from build123d import *

# Parameters (mm, degrees)
EXTRUDE_1_DEPTH = 50


with BuildPart() as part:
    # 草图1 → 凸台-拉伸1 (new body)
    with BuildSketch(Plane(origin=(0, 0, 0), x_dir=(0, 0, -1), z_dir=(1, 0, 0))):
        with BuildLine():
            Line((-5.14957074, -13.70467014), (-4.14957074, -13.70467014))
            Line((-4.14957074, -13.70467014), (-4.14957074, -12.70467014))
            Line((-4.14957074, -12.70467014), (-8.29957074, -12.70467014))
            Line((-8.29957074, -12.70467014), (-8.29957074, -9.3688837))
            Line((-8.29957074, -9.3688837), (-4.43535718, -5.50467014))
            Line((-4.43535718, -5.50467014), (4.3362157, -5.50467014))
            Line((4.3362157, -5.50467014), (8.20042926, -9.3688837))
            Line((8.20042926, -9.3688837), (8.20042926, -12.70467014))
            Line((8.20042926, -12.70467014), (4.05042926, -12.70467014))
            Line((4.05042926, -12.70467014), (4.05042926, -13.70467014))
            Line((4.05042926, -13.70467014), (5.05042926, -13.70467014))
            Line((5.05042926, -13.70467014), (5.05042926, -14.70467014))
            Line((5.05042926, -14.70467014), (12.45042926, -14.70467014))
            ThreePointArc((12.45042926, -14.70467014), (14.218196213, -13.972437093), (14.95042926, -12.20467014))
            Line((14.95042926, -12.20467014), (14.95042926, -4.80467014))
            Line((14.95042926, -4.80467014), (13.95042926, -4.80467014))
            Line((13.95042926, -4.80467014), (13.95042926, -3.80467014))
            Line((13.95042926, -3.80467014), (12.95042926, -3.80467014))
            Line((12.95042926, -3.80467014), (12.95042926, -7.95467014))
            Line((12.95042926, -7.95467014), (9.61464282, -7.95467014))
            Line((9.61464282, -7.95467014), (5.75042926, -4.09045658))
            Line((5.75042926, -4.09045658), (5.75042926, 4.6811163))
            Line((5.75042926, 4.6811163), (9.61464282, 8.54532986))
            Line((9.61464282, 8.54532986), (12.95042926, 8.54532986))
            Line((12.95042926, 8.54532986), (12.95042926, 4.39532986))
            Line((12.95042926, 4.39532986), (13.95042926, 4.39532986))
            Line((13.95042926, 4.39532986), (13.95042926, 5.39532986))
            Line((13.95042926, 5.39532986), (14.95042926, 5.39532986))
            Line((14.95042926, 5.39532986), (14.95042926, 12.79532986))
            ThreePointArc((14.95042926, 12.79532986), (14.218196213, 14.563096813), (12.45042926, 15.29532986))
            Line((12.45042926, 15.29532986), (5.05042926, 15.29532986))
            Line((5.05042926, 15.29532986), (5.05042926, 14.29532986))
            Line((5.05042926, 14.29532986), (4.05042926, 14.29532986))
            Line((4.05042926, 14.29532986), (4.05042926, 13.29532986))
            Line((4.05042926, 13.29532986), (8.20042926, 13.29532986))
            Line((8.20042926, 13.29532986), (8.20042926, 9.95954342))
            Line((8.20042926, 9.95954342), (4.3362157, 6.09532986))
            Line((4.3362157, 6.09532986), (-4.43535718, 6.09532986))
            Line((-4.43535718, 6.09532986), (-8.29957074, 9.95954342))
            Line((-8.29957074, 9.95954342), (-8.29957074, 13.29532986))
            Line((-8.29957074, 13.29532986), (-4.14957074, 13.29532986))
            Line((-4.14957074, 13.29532986), (-4.14957074, 14.29532986))
            Line((-4.14957074, 14.29532986), (-5.14957074, 14.29532986))
            Line((-5.14957074, 14.29532986), (-5.14957074, 15.29532986))
            Line((-5.14957074, 15.29532986), (-12.54957074, 15.29532986))
            ThreePointArc((-12.54957074, 15.29532986), (-14.317337693, 14.563096813), (-15.04957074, 12.79532986))
            Line((-15.04957074, 12.79532986), (-15.04957074, 5.39532986))
            Line((-15.04957074, 5.39532986), (-14.04957074, 5.39532986))
            Line((-14.04957074, 5.39532986), (-14.04957074, 4.39532986))
            Line((-14.04957074, 4.39532986), (-13.04957074, 4.39532986))
            Line((-13.04957074, 4.39532986), (-13.04957074, 8.54532986))
            Line((-13.04957074, 8.54532986), (-9.7137843, 8.54532986))
            Line((-9.7137843, 8.54532986), (-5.84957074, 4.6811163))
            Line((-5.84957074, 4.6811163), (-5.84957074, -4.09045658))
            Line((-5.84957074, -4.09045658), (-9.7137843, -7.95467014))
            Line((-9.7137843, -7.95467014), (-13.04957074, -7.95467014))
            Line((-13.04957074, -7.95467014), (-13.04957074, -3.80467014))
            Line((-13.04957074, -3.80467014), (-14.04957074, -3.80467014))
            Line((-14.04957074, -3.80467014), (-14.04957074, -4.80467014))
            Line((-14.04957074, -4.80467014), (-15.04957074, -4.80467014))
            Line((-15.04957074, -4.80467014), (-15.04957074, -12.20467014))
            ThreePointArc((-15.04957074, -12.20467014), (-14.317337693, -13.972437093), (-12.54957074, -14.70467014))
            Line((-12.54957074, -14.70467014), (-5.14957074, -14.70467014))
            Line((-5.14957074, -14.70467014), (-5.14957074, -13.70467014))
        make_face()
        with BuildLine():
            Line((-10.04957074, 9.79532986), (-13.04957074, 9.79532986))
            ThreePointArc((-13.04957074, 9.79532986), (-13.403124131, 9.941776469), (-13.54957074, 10.29532986))
            Line((-13.54957074, 10.29532986), (-13.54957074, 13.29532986))
            ThreePointArc((-13.54957074, 13.29532986), (-13.403124131, 13.648883251), (-13.04957074, 13.79532986))
            Line((-13.04957074, 13.79532986), (-10.04957074, 13.79532986))
            ThreePointArc((-10.04957074, 13.79532986), (-9.696017349, 13.648883251), (-9.54957074, 13.29532986))
            Line((-9.54957074, 13.29532986), (-9.54957074, 10.29532986))
            ThreePointArc((-9.54957074, 10.29532986), (-9.696017349, 9.941776469), (-10.04957074, 9.79532986))
        make_face(mode=Mode.SUBTRACT)
        with BuildLine():
            Line((-10.04957074, -13.20467014), (-13.04957074, -13.20467014))
            ThreePointArc((-13.04957074, -13.20467014), (-13.403124131, -13.058223531), (-13.54957074, -12.70467014))
            Line((-13.54957074, -12.70467014), (-13.54957074, -9.70467014))
            ThreePointArc((-13.54957074, -9.70467014), (-13.403124131, -9.351116749), (-13.04957074, -9.20467014))
            Line((-13.04957074, -9.20467014), (-10.04957074, -9.20467014))
            ThreePointArc((-10.04957074, -9.20467014), (-9.696017349, -9.351116749), (-9.54957074, -9.70467014))
            Line((-9.54957074, -9.70467014), (-9.54957074, -12.70467014))
            ThreePointArc((-9.54957074, -12.70467014), (-9.696017349, -13.058223531), (-10.04957074, -13.20467014))
        make_face(mode=Mode.SUBTRACT)
        with BuildLine():
            Line((12.95042926, 9.79532986), (9.95042926, 9.79532986))
            ThreePointArc((9.95042926, 9.79532986), (9.596875869, 9.941776469), (9.45042926, 10.29532986))
            Line((9.45042926, 10.29532986), (9.45042926, 13.29532986))
            ThreePointArc((9.45042926, 13.29532986), (9.596875869, 13.648883251), (9.95042926, 13.79532986))
            Line((9.95042926, 13.79532986), (12.95042926, 13.79532986))
            ThreePointArc((12.95042926, 13.79532986), (13.303982651, 13.648883251), (13.45042926, 13.29532986))
            Line((13.45042926, 13.29532986), (13.45042926, 10.29532986))
            ThreePointArc((13.45042926, 10.29532986), (13.303982651, 9.941776469), (12.95042926, 9.79532986))
        make_face(mode=Mode.SUBTRACT)
        with BuildLine():
            Line((13.45042926, -9.70467014), (13.45042926, -12.70467014))
            ThreePointArc((13.45042926, -12.70467014), (13.303982651, -13.058223531), (12.95042926, -13.20467014))
            Line((12.95042926, -13.20467014), (9.95042926, -13.20467014))
            ThreePointArc((9.95042926, -13.20467014), (9.596875869, -13.058223531), (9.45042926, -12.70467014))
            Line((9.45042926, -12.70467014), (9.45042926, -9.70467014))
            ThreePointArc((9.45042926, -9.70467014), (9.596875869, -9.351116749), (9.95042926, -9.20467014))
            Line((9.95042926, -9.20467014), (12.95042926, -9.20467014))
            ThreePointArc((12.95042926, -9.20467014), (13.303982651, -9.351116749), (13.45042926, -9.70467014))
        make_face(mode=Mode.SUBTRACT)
        with BuildLine():
            Line((-4.07998961, 3.61864195), (-3.37288283, 4.32574873))
            Line((-3.37288283, 4.32574873), (-2.07404174, 3.02690764))
            ThreePointArc((-2.07404174, 3.02690764), (-0.04957074, 3.69532986), (1.97490026, 3.02690764))
            Line((1.97490026, 3.02690764), (3.27374135, 4.32574873))
            Line((3.27374135, 4.32574873), (3.98084813, 3.61864195))
            Line((3.98084813, 3.61864195), (2.68200704, 2.31980086))
            ThreePointArc((2.68200704, 2.31980086), (3.35042926, 0.29532986), (2.68200704, -1.72914114))
            Line((2.68200704, -1.72914114), (3.98084813, -3.02798223))
            Line((3.98084813, -3.02798223), (3.27374135, -3.73508901))
            Line((3.27374135, -3.73508901), (1.97490026, -2.43624792))
            ThreePointArc((1.97490026, -2.43624792), (-0.04957074, -3.10467014), (-2.07404174, -2.43624792))
            Line((-2.07404174, -2.43624792), (-3.37288283, -3.73508901))
            Line((-3.37288283, -3.73508901), (-4.07998961, -3.02798223))
            Line((-4.07998961, -3.02798223), (-2.78114852, -1.72914114))
            ThreePointArc((-2.78114852, -1.72914114), (-3.44957074, 0.29532986), (-2.78114852, 2.31980086))
            Line((-2.78114852, 2.31980086), (-4.07998961, 3.61864195))
        make_face(mode=Mode.SUBTRACT)
    extrude(amount=-EXTRUDE_1_DEPTH)


solid = part.part
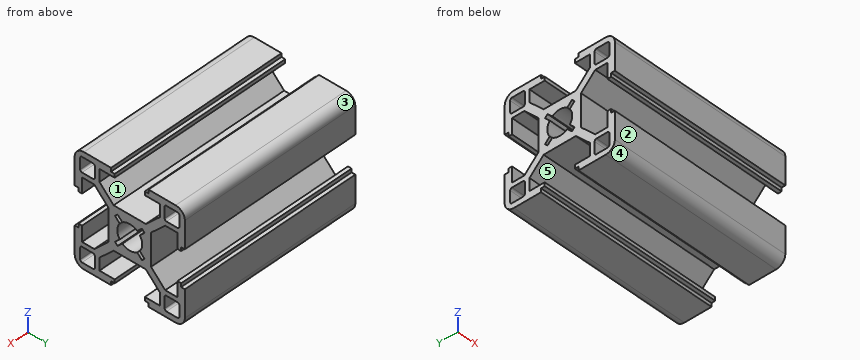
Model file for the job. Use its own axes, mm. Face numbers are marked on the shaded views. A direction names the side the tool comes from. Give positions to 0.01 mm unless a question says otherwise; leave off trailing zeros. Loops run counter-clockwise (first coordinate to the right, second up) from the corner with the lowest first, then second, coordinate; pieces in that order, holes last. Notation, with made-up numbers: (-6.75, 11) - (49.25, 11) arc R23 ccw to (49.25, 27) - close; hole circle Ø4 at (-23, 39.25). An arc over 180 degrees is marked (long way). Use one line per item in the form item = value.
(1) Pull direction Z, two halves, no side cores. Call the marked faces 3, 4 and 5: pulls with the +Z half, pulls with the -Z half, needs draft (parallel to the pull), parting line crosses it, or undercut.
Determined:
face_3 = pulls with the +Z half
face_4 = pulls with the -Z half
face_5 = undercut
(2) Cut at B-B (z = -0.5). Give the cut face in (x, y).
Determined:
outline = (-50, -5.5) - (0, -5.5) - (0, -3.06) - (-50, -3.06) - close; (-50, 3.65) - (0, 3.65) - (0, 6.1) - (-50, 6.1) - close
(3) Cut at C-C (x = -29). Count the separate pieces of the cut face and the enclosed holes in it, then the cut area to 3 significant figures.
Determined:
separate_pieces = 1
enclosed_holes = 5
area = 299 mm^2
(4) Drill centre lines: L1, parallel to Z at x = -36, y = 10.5; L2, parallel to Y at x = -9.5, z = 12.75; L3, parallel to Z at x = -12.5, y = 7. Where is each one in solid material? Low to high.
Determined:
L1 = -14.95 to -13.45, -9.45 to -8.2, 8.3 to 9.55, 13.55 to 15.05
L2 = -14.7 to -13.2, -9.2 to -7.95, 8.55 to 9.8, 13.8 to 15.29
L3 = -14.95 to -12.95, -8.07 to -5.24, 5.34 to 8.17, 13.05 to 15.05
(5) Drop flat-ended pins along their axis: P1, Ø0.8, axis at x = -32.5, z = -13.5, coming from the +Y side; P2, Ø3, axis at y = 4.5, z = 3, coming from the +X side; P3, Ø4.5, axis at x = -13, y = 2.5, coming from the -Z side; P4, Ø5, axis at x = -18.5, z = -2, coming from the +Y side. Give the stop position or say it passes through.
Determined:
P1 = 15.21
P2 = 0
P3 = -13.95
P4 = 14.3
(6) 3-axis set-ups, long thin cutter, end or side, ignore diameter. For the marked faces 1 and 2: which of +Z, -Z, +X, -X, +Y, -Y reach the whole face in a straight line?
Determined:
face_1 = +X, -X
face_2 = +Z, -Z, +X, -X, -Y
(7) Cut at A-A (y = 11). Give the cut face in (x, z).
Determined:
outline = (-50, -14.95) - (0, -14.95) - (0, -13.45) - (-50, -13.45) - close; (-50, -9.45) - (0, -9.45) - (0, -8.2) - (-50, -8.2) - close; (-50, 8.3) - (0, 8.3) - (0, 9.55) - (-50, 9.55) - close; (-50, 13.55) - (0, 13.55) - (0, 15.05) - (-50, 15.05) - close
